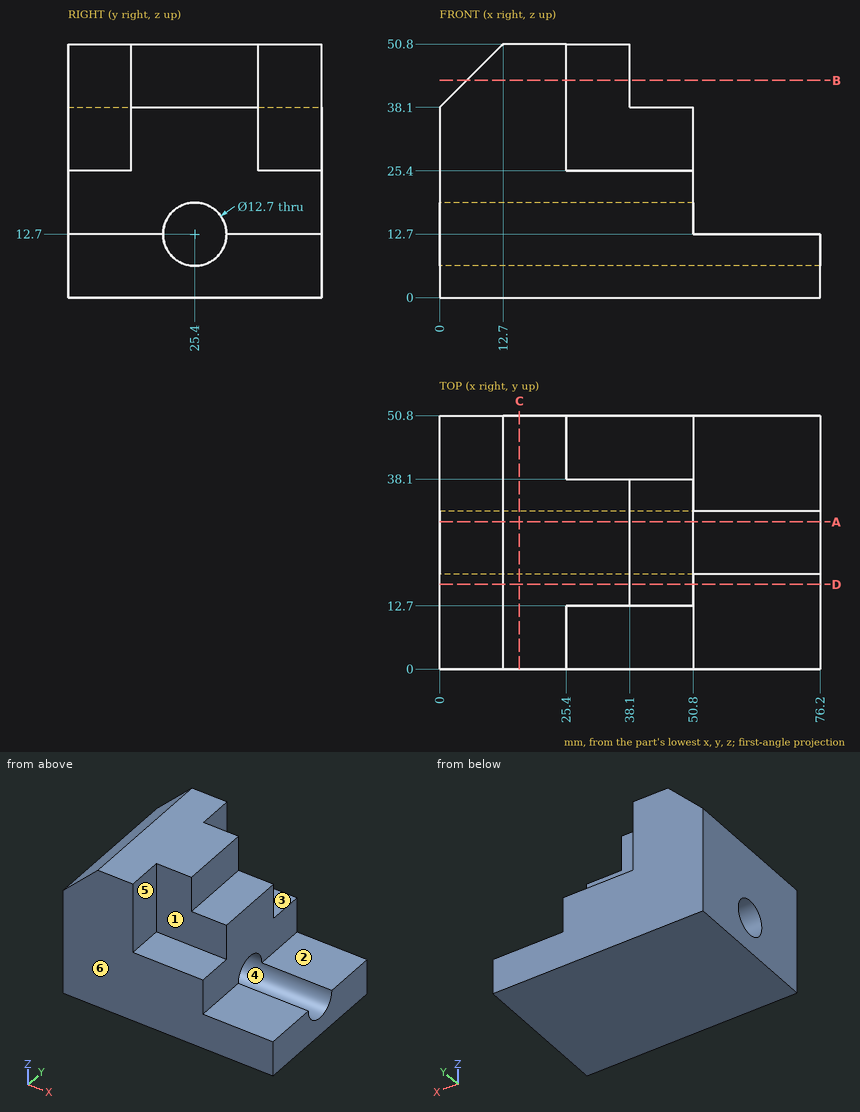
Geometry: see drawing. Coordinates: mm, zero at the bounding-box minimum. A direction names the side the tool comes from. Give positions to 0.01 mm unless a question says otherwise; leave off trailing zeros. Loops run counter-clockwise (first coordinate to the right, second up) from the corner with the lowest first, then second, coordinate; pieces in that order, holes last. Notation, with made-up numbers: (-4, 53.25) -> (13, 53.25) arc R26 ccw to (13, 69.25) -> close; hole circle Ø11 at (23, 24). An arc over 180 degrees is marked (long way). Use one line per item in the form item = value.
Item 1: Draft query along Y for the marked faces 4, 5 and 6. Return one class per face: pulls with the +Y half, pulls with the -Y half, needs draft (parallel to the pull), parting line crosses it, or undercut.
A:
face_4 = undercut
face_5 = needs draft
face_6 = pulls with the -Y half
Item 2: Section query C-C on x = 16. Output: boundary loops of the cut face in (y, z), and give its area (3 significant figures).
A:
outline = (0, 0) -> (50.8, 0) -> (50.8, 50.8) -> (0, 50.8) -> close; hole circle Ø12.7 at (25.4, 12.7)
area = 2,450 mm^2
Item 3: Access query for the marked faces 1, 2 and 3. Directions: +Z, -Z, +X, -X, +Y, -Y. A direction counts if a zero-diameter tool reaches every point of the face in a straight line with its end or side. Return the directions, or none.
A:
face_1 = +Z, +X, -Y
face_2 = +Z, +X, +Y, -Y
face_3 = +Z, +X, +Y
Item 4: Line query: probe 1 along Y at (x, z) = (39.5, 12.7); probe 2 along Z at (x, y) = (16.5, 25.4); probe 3 along X at (y, z) = (4, 29). Output: solid intervals per line, ascending.
A:
probe_1 = 0 to 19.05, 31.75 to 50.8
probe_2 = 0 to 6.35, 19.05 to 50.8
probe_3 = 0 to 25.4
Item 5: Section query A-A on y = 29.5. Output: boundary loops of the cut face in (x, z), and give its area (3 significant figures).
A:
outline = (0, 0) -> (76.2, 0) -> (76.2, 7.85) -> (0, 7.85) -> close; (0, 17.55) -> (50.8, 17.55) -> (50.8, 38.1) -> (38.1, 38.1) -> (38.1, 50.8) -> (12.7, 50.8) -> (0, 38.1) -> close
area = 2,050 mm^2
Item 6: Section query B-B on z = 43.5. Output: boundary loops of the cut face in (x, y), and give its area (3 significant figures).
A:
outline = (5.4, 0) -> (25.4, 0) -> (25.4, 12.7) -> (38.1, 12.7) -> (38.1, 38.1) -> (25.4, 38.1) -> (25.4, 50.8) -> (5.4, 50.8) -> close
area = 1,340 mm^2
Item 7: Pin query (flat end, axial travel): P1, Ø6.5, axis at x = 46.5, y = 26, coming from the +Z side; P2, Ø20.5, axis at x = 44, z = 40.5, coming from the -Y side; P3, Ø20.5, axis at y = 37.5, z = 29, coming from the +X side. Return the tip coordinate at first contact, or that it passes through.
A:
P1 = 38.1
P2 = 12.7
P3 = 50.8
Item 8: Section query D-D on y = 17. Output: boundary loops of the cut face in (x, z), and give its area (3 significant figures).
A:
outline = (0, 0) -> (76.2, 0) -> (76.2, 12.7) -> (50.8, 12.7) -> (50.8, 38.1) -> (38.1, 38.1) -> (38.1, 50.8) -> (12.7, 50.8) -> (0, 38.1) -> close
area = 2,660 mm^2
